Design review of the part built by this model. Coordinates are the model's own, in mm. Coordinates: 2 decimals unless noted, no trailing zeros. Loops run counter-clockwise (first coordinate to the right, second up) from the corner with the lowest first, then second, coordinate; pieces in that order, holes last. Notation, with made-up numbers: (52, 76) -> (92, 76) arc R22 cw to (92, 103) -> close; hole circle Ø2 at (31, 0.5). An arc over 180 degrees is marked (long way). Use a Markdown table: item, result. Add a question column.
Q1. Clearance check with flat-ended pins moving along their axes: pin 1 Ø5 at (x, z) = (1.5, -2) entering from -Y; pin 2 Ø1.3 at (y, z) = (35, -18.5) entering from +X. State where each tip first meets the part, or that it passes through.
Q2. For probe 1 along Z at (x, y) = (4, -68.5); probe 2 along Z at (x, y) = (7.5, 7.5); probe 3 along Y at (x, z) = (4, -15.5), list the stretches that pass through material, from the lowest coordinate up.
Q3. Take a section at A-A on y = 53.5. Write out the cut boundary in (x, z), plus the area to 3 significant figures.
Q4. Take a section at B-B on x = 6.5. Write out the cut boundary in (y, z).
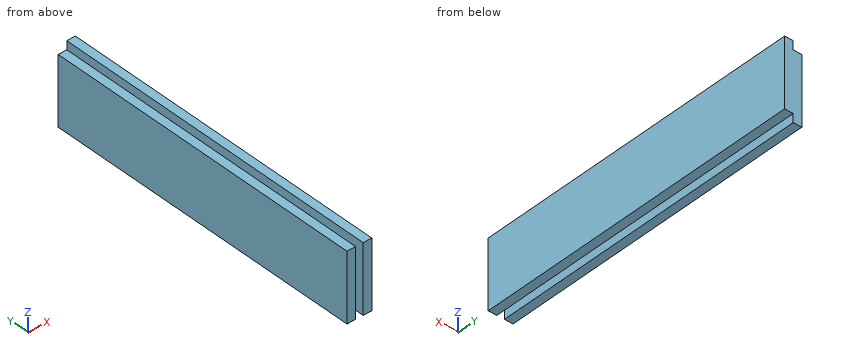
from build123d import *

# Parameters (mm, degrees)
F0_W     = 174
F0_H     = 40.5
F1_DEPTH = 9
F2_W     = 4.5
F2_H     = 174
F3_DEPTH = 4.5
F4_W     = 4.5
F4_H     = 4.5
F5_DEPTH = 36
F6_W     = 4.5
F6_H     = 4.5
F7_DEPTH = 4.5
F8_W     = 4.5
F8_H     = 169.5
F9_DEPTH = 4.5


with BuildPart() as f1:
    # F0 (on Right) → F1 (new body)
    with BuildSketch(Plane.YZ):
        Rectangle(F0_W, F0_H)
    extrude(amount=F1_DEPTH)

    # F2 (on face) → F3 (cut)
    with BuildSketch(Plane.XY.offset(20.25)):
        with Locations((2.25, 0)):
            Rectangle(F2_W, F2_H)
    extrude(amount=-F3_DEPTH, mode=Mode.SUBTRACT)

    # F4 (on face) → F5 (cut, through all)
    with BuildSketch(Plane.XY.offset(15.75)):
        with Locations((2.25, -84.75)):
            Rectangle(F4_W, F4_H)
    extrude(amount=-F5_DEPTH, mode=Mode.SUBTRACT)

    # F6 (on face) → F7 (cut)
    with BuildSketch(Plane(origin=(0, 0, -20.25), x_dir=(1, 0, 0), z_dir=(0, 0, -1))):
        with Locations((6.75, 84.75)):
            Rectangle(F6_W, F6_H)
    extrude(amount=-F7_DEPTH, mode=Mode.SUBTRACT)

    # F8 (on face) → F9 (cut)
    with BuildSketch(Plane(origin=(0, 0, -20.25), x_dir=(1, 0, 0), z_dir=(0, 0, -1))):
        with Locations((6.75, -2.25)):
            Rectangle(F8_W, F8_H)
    extrude(amount=-F9_DEPTH, mode=Mode.SUBTRACT)


solid = f1.part
Answer list:
| question | item | result |
|---|---|---|
| 1 | pin 1 | y = -82.5 |
| 1 | pin 2 | x = 4.5 |
| 2 | probe 1 | -20.25 to 15.75 |
| 2 | probe 2 | -15.75 to 20.25 |
| 2 | probe 3 | -82.5 to 87 |
| 3 | outline | (0, -20.25) -> (4.5, -20.25) -> (4.5, -15.75) -> (9, -15.75) -> (9, 20.25) -> (4.5, 20.25) -> (4.5, 15.75) -> (0, 15.75) -> close |
| 3 | area | 324 mm² |
| 4 | outline | (-87, -15.75) -> (87, -15.75) -> (87, 20.25) -> (-87, 20.25) -> close |
